Geometry check sheet. Reference: drawing and pictorial views, mm from the part's lowest x, y, z. Coordinates: 2 decimals unless noted, no trailing zeros. Loops run counter-clockwise (first coordinate to the right, second up) from the corner with the lowest first, then second, coordinate; pieces in that order, holes last.
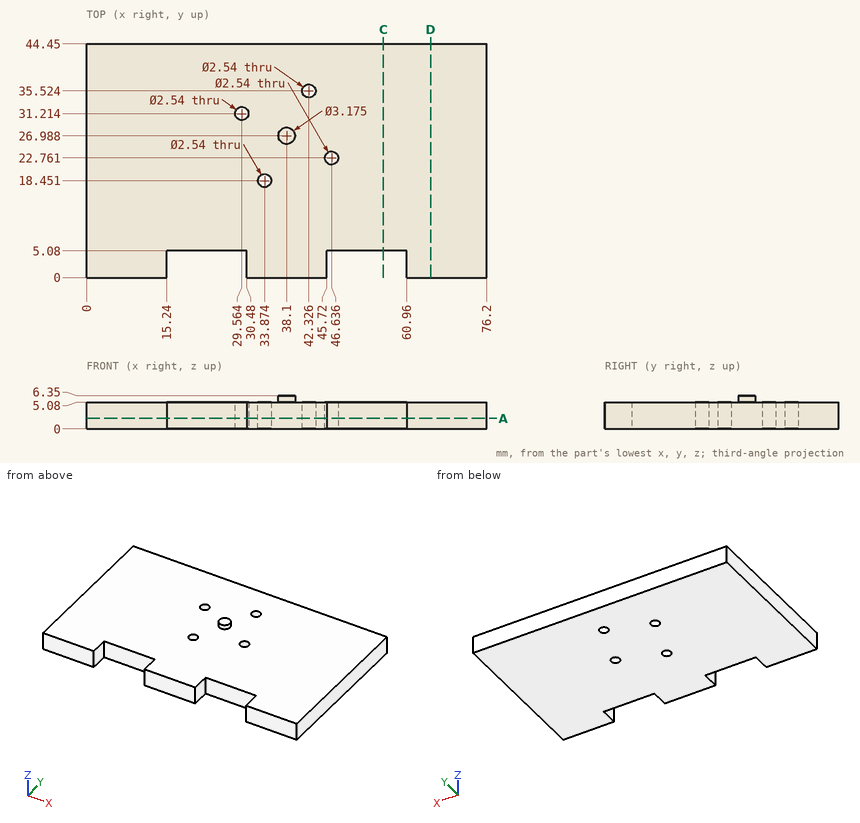
1) Section check C-C on x = 56.5. Record the cut outline in (y, z), and give its area (3 significant figures).
Data:
outline: (5.08, 0) - (44.45, 0) - (44.45, 5.08) - (5.08, 5.08) - close
area: 200 mm2
2) Section check D-D on x = 65.5. Record the cut outline in (y, z).
Data:
outline: (0, 0) - (44.45, 0) - (44.45, 5.08) - (0, 5.08) - close
3) Depth check by flat-ended pin: pin 1 (13.5 mm diameter, centred on x = 29, y = 30.5, fed in from +Z); pin 2 (1 mm diameter, centred on x = 67, z = 1, fed in from -Y); pin 3 (1.5 mm diameter, centred on x = 27.5, z = 1.5, fed in from -Y). Enter the tip coordinate at first touch or a pass-through.
Data:
pin 1: stops at z = 5.08
pin 2: stops at y = 0
pin 3: stops at y = 5.08
4) Material ranges on probe 1 along X at (y, z) = (5, 4.5); probe 2 along Y at (x, z) = (52, 4.5); probe 3 along Z at (x, y) = (3, 37.5), recorded low to high.
Data:
probe 1: x = 0 to 15.24, 30.48 to 45.72, 60.96 to 76.2
probe 2: y = 5.08 to 44.45
probe 3: z = 0 to 5.08
5) Section check A-A on z = 2. Record the cut outline in (x, y).
Data:
outline: (0, 0) - (15.24, 0) - (15.24, 5.08) - (30.48, 5.08) - (30.48, 0) - (45.72, 0) - (45.72, 5.08) - (60.96, 5.08) - (60.96, 0) - (76.2, 0) - (76.2, 44.45) - (0, 44.45) - close; hole circle Ø2.54 at (29.56, 31.21); hole circle Ø2.54 at (33.87, 18.45); hole circle Ø2.54 at (42.33, 35.52); hole circle Ø2.54 at (46.64, 22.76)
